Read the model definition and answer for the solid it produces. Units are mm, in the model's axes. Coordinates: 2 decimals unless noted, no trailing zeros. Write each loop counter-clockwise with the first axis right and the second up, starting at its lowest first coordinate (ties: lowest second). Pieces come first, ordered by that corner, then holes.
1) Find the intervals of material crossed by line 1 (Z direction, x = 0, y = -6); line 2 (X direction, y = -32.5, z = 23.5); line 3 (X direction, y = 31, z = -12), in increasing order.
2) The part is cut by section B-B (z = 0). Determine the outline of the cut face in (x, y), then the cut area to 3 significant figures.
3) The part is cut by section C-C (y = -14). Determine the outline of the cut face in (x, z).
4) The part is cut by section A-A (x = 0). Determine the outline of the cut face in (y, z).
5) Determine the mould class of faces 1 (the face through (-125.19, -0.53, -61.59)), 2 (the face through (-127, -1, -1)), 3 (the face through (-30.235, -0.533, -23.183)) for opening direction Z: +Z half, -Z half, draft (parallel to the pull), parting line (faces both ways), or undercut.
from build123d import *

# Parameters (mm, degrees)
F0_W     = 254
F0_H     = 127
F1_DEPTH = 38.1
F2_R     = 6.35
F3_R     = 38.1
F4_DEPTH = 76.201


with BuildPart() as f1:
    # F0 (on Front) → F1 (new body, symmetric)
    with BuildSketch(Plane.XZ):
        Rectangle(F0_W, F0_H)
    extrude(amount=F1_DEPTH, both=True)

    # F2
    f2_edges = [f1.edges().sort_by_distance(p)[0] for p in [
        (-127, 0, 63.5),
        (127, 0, 63.5),
        (-127, 0, -63.5),
        (127, 0, -63.5),
    ]]
    fillet(f2_edges, radius=F2_R)

    # F3 (on face) → F4 (cut, through all)
    with BuildSketch(Plane.XZ.offset(38.1)):
        Circle(F3_R)
    extrude(amount=-F4_DEPTH, mode=Mode.SUBTRACT)


solid = f1.part
Reported:
1. line 1: z = -63.5 to -38.1, 38.1 to 63.5
1. line 2: x = -127 to -29.99, 29.99 to 127
1. line 3: x = -127 to -36.16, 36.16 to 127
2. outline: (-127, -38.1) - (-38.1, -38.1) - (-38.1, 38.1) - (-127, 38.1) - close; (38.1, -38.1) - (127, -38.1) - (127, 38.1) - (38.1, 38.1) - close
2. area: 13,500 mm2
3. outline: (-127, -57.15) arc R6.35 ccw to (-120.65, -63.5) - (120.65, -63.5) arc R6.35 ccw to (127, -57.15) - (127, 57.15) arc R6.35 ccw to (120.65, 63.5) - (-120.65, 63.5) arc R6.35 ccw to (-127, 57.15) - close; hole circle Ø76.2 at (0, 0)
4. outline: (-38.1, -63.5) - (38.1, -63.5) - (38.1, -38.1) - (-38.1, -38.1) - close; (-38.1, 38.1) - (38.1, 38.1) - (38.1, 63.5) - (-38.1, 63.5) - close
5. face 1: -Z half
5. face 2: draft
5. face 3: undercut
